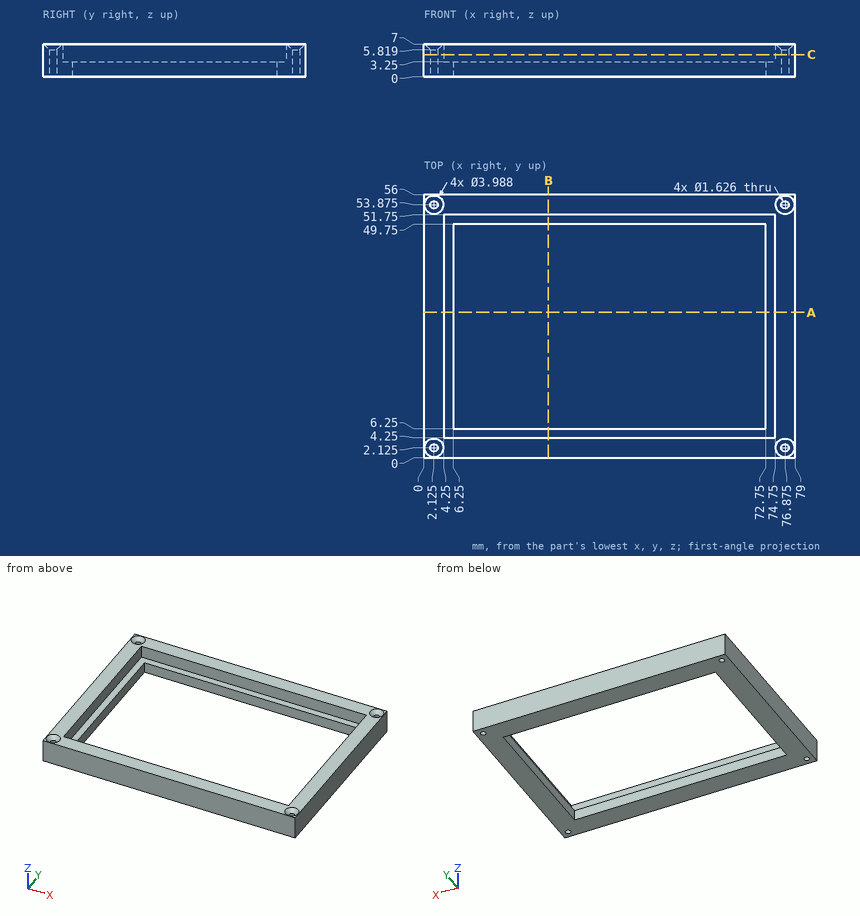
Source: three-view drawing plus pictorial views. Frame: mm from the lowest corner of the part. Round coordinates to 2 decimals unless told otherwise and drop trailing zeros. Loops run counter-clockwise (first coordinate to the right, second up) from the corner with the lowest first, then second, coordinate; pieces in that order, holes last. Notation, with made-up numbers: M 3,69 L 38,69 A20 ccw 38,77 Z; hole C 62,72 d8. An arc over 180 degrees is marked long. Answer as CSV lines item,"result".
Q1. Cut plane C-C (z = 4.75). Count the separate pieces of the cut face and the enclosed holes in it, plus the area to 3 significant figures.
Verdict:
separate pieces,"1"
enclosed holes,"5"
area,"1,070 mm^2"
Q2. Cut plane A-A (y = 31). Return the cut outline in (x, z), plus the area to 3 significant figures.
Verdict:
outline,"M 0,0 L 6.25,0 L 6.25,3.25 L 4.25,3.25 L 4.25,7 L 0,7 Z; M 72.75,0 L 79,0 L 79,7 L 74.75,7 L 74.75,3.25 L 72.75,3.25 Z"
area,"72.5 mm^2"
Q3. Line query: line 1 along X through (y, z) = (19, 4); line 2 along X through (y, z) = (17.5, 2.5); line 3 along Y through (x, z) = (34, 6). Output: solid intervals per line, ascending.
Verdict:
line 1,"x = 0 to 4.25, 74.75 to 79"
line 2,"x = 0 to 6.25, 72.75 to 79"
line 3,"y = 0 to 4.25, 51.75 to 56"
Q4. Contact query for flat-ended pins moving along their axis: pin 1 (1 mm diameter, centred on x = 2.125, y = 53.875, fed in from +Z); pin 2 (12 mm diameter, centred on x = 61.5, y = 11, fed in from +Z); pin 3 (2 mm diameter, centred on x = 2.125, y = 2.125, fed in from +Z) (1 decimal). Output: stop coordinate, or through.
Verdict:
pin 1,"passes through"
pin 2,"stops at z = 3.25"
pin 3,"stops at z = 6"
Q5. Cut plane B-B (x = 26.5). Return the cut outline in (y, z).
Verdict:
outline,"M 0,0 L 6.25,0 L 6.25,3.25 L 4.25,3.25 L 4.25,7 L 0,7 Z; M 49.75,0 L 56,0 L 56,7 L 51.75,7 L 51.75,3.25 L 49.75,3.25 Z"
